The drawing under review shows one solid part. Ordinate dimensions are in mm from its lowest x, y, z. A direction names the side the tool comes from. Coordinates: 2 decimals unless noted, no trailing zeros. Write each loop counter-clockwise with the first axis right and the second up, starting at its lowest first coordinate (ties: lowest second). Pieces come first, ordered by that corner, then holes. Notation, with made-up numbers: (80.5, 22.25) - (111.5, 22.25) arc R23 cw to (111.5, 56.25) - close; hole circle Ø11 at (16, -19.5). An arc over 180 degrees is marked (long way). Use a Markdown table: item, result.
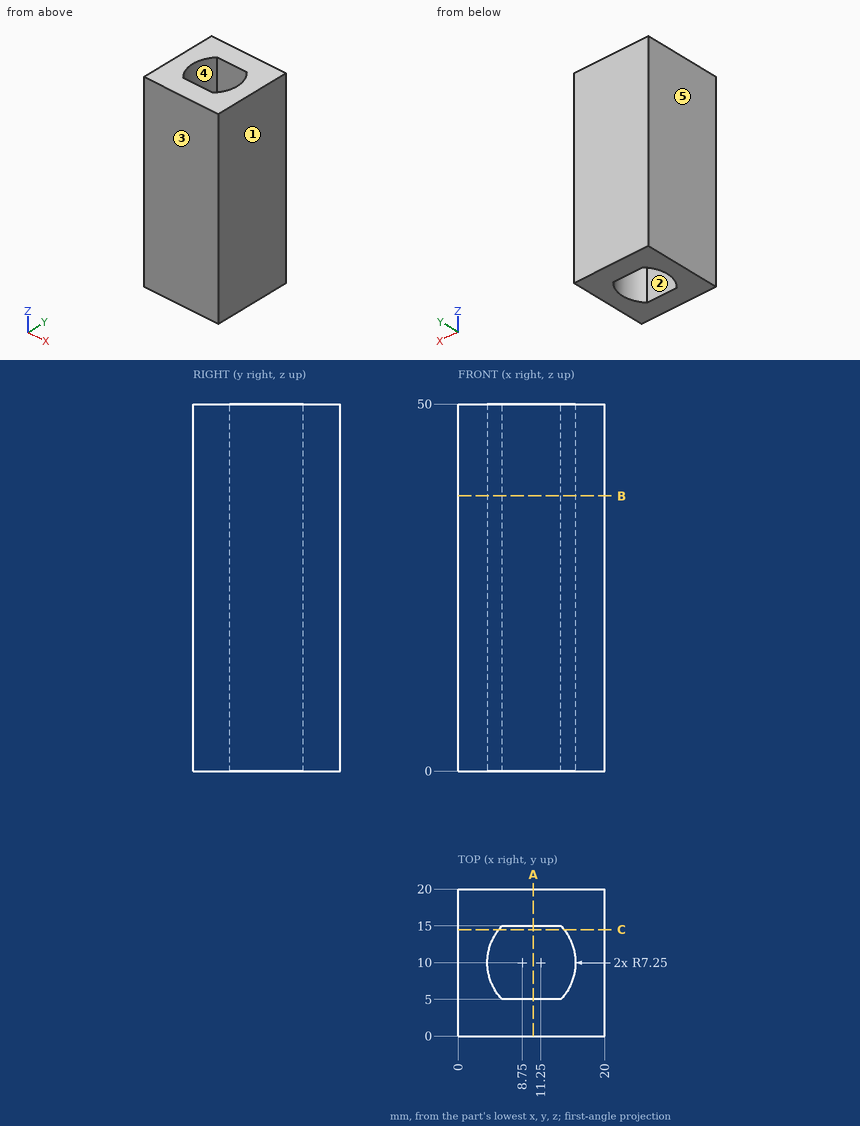
(1) For pin 1 (12 mm diameter, centred on x = 8, y = 5.5, fed in from -Z), flat-tipped, find the tip position at first contact; note if it passes through.
Determined:
| item | result |
|---|---|
| pin 1 | z = 0 |
(2) Draft analysis for pull direction X (two halves, no side actions). For the marked faces 3, 4 and 5, state which applies: +X half, -X half, draft (parallel to the pull), parting line (faces both ways), or undercut.
Determined:
| item | result |
|---|---|
| face 3 | draft |
| face 4 | undercut |
| face 5 | -X half |
(3) Take a section at C-C on y = 14.5. Write out the cut boundary in (x, z), and give its area (3 significant figures).
Determined:
| item | result |
|---|---|
| outline | (0, 0) - (5.57, 0) - (5.57, 50) - (0, 50) - close; (14.43, 0) - (20, 0) - (20, 50) - (14.43, 50) - close |
| area | 557 mm2 |
(4) For L1, parallel to Y at x = 6.5, z = 45; L2, parallel to X at y = 10, z = 17; L3, parallel to X at y = 8.5, z = 10, list the stretches that pass through material, from the lowest coordinate up. Write a range as from..to.
Determined:
| item | result |
|---|---|
| L1 | 0..5, 15..20 |
| L2 | 0..4, 16..20 |
| L3 | 0..4.16, 15.84..20 |
(5) Machinability: for the marked faces 1 and 2, which of the approach directions +Z, -Z, +X, -X, +Y, -Y give a long, thin tool a straight path to every point of the face, cutting with its end or side? Answer none if there is none.
Determined:
| item | result |
|---|---|
| face 1 | +Z, -Z, +X, +Y, -Y |
| face 2 | +Z, -Z |
(6) Take a section at A-A on x = 10.25. Write out the cut boundary in (y, z), and give its area (3 significant figures).
Determined:
| item | result |
|---|---|
| outline | (0, 0) - (5, 0) - (5, 50) - (0, 50) - close; (15, 0) - (20, 0) - (20, 50) - (15, 50) - close |
| area | 500 mm2 |
(7) Take a section at B-B on z = 37.5. Write out the cut boundary in (x, y), and give its area (3 significant figures).
Determined:
| item | result |
|---|---|
| outline | (0, 0) - (20, 0) - (20, 20) - (0, 20) - close; hole (6, 5) - (14, 5) arc R7.25 ccw to (14, 15) - (6, 15) arc R7.25 ccw to start |
| area | 292 mm2 |
